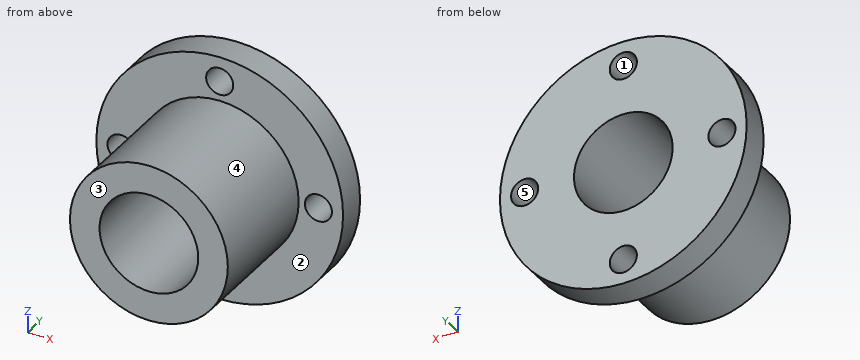
```python
from build123d import *

# Parameters (mm, degrees)
F0_R     = 25
F1_DEPTH = 6
F2_R     = 16
F3_DEPTH = 25
F4_R     = 2.75
F5_DEPTH = 31.001
F7_D     = 20


with BuildPart() as f1:
    # F0 (on Front) → F1 (new body)
    with BuildSketch(Plane.XZ):
        Circle(F0_R)
    extrude(amount=F1_DEPTH)

    # F2 (on face) → F3 (join)
    with BuildSketch(Plane.XZ.offset(6)):
        Circle(F2_R)
    extrude(amount=F3_DEPTH)

    # F4 (on face) → F5 (cut, through all)
    with BuildSketch(Plane(origin=(0, 0, 0), x_dir=(-1, 0, 0), z_dir=(0, 1, 0))):
        with Locations((0, 20)):
            Circle(F4_R)
        with Locations((-20, 0)):
            Circle(F4_R)
        with Locations((20, 0)):
            Circle(F4_R)
        with Locations((0, -20)):
            Circle(F4_R)
    extrude(amount=-F5_DEPTH, mode=Mode.SUBTRACT)

    # F7 (through all)
    with Locations(Plane(origin=(0, 0, 0), x_dir=(-1, 0, 0), z_dir=(0, 1, 0))):
        with Locations((0, 0)):
            Hole(F7_D / 2)


solid = f1.part
```
CAD build for the part. Positions are in the model's coordinates, mm. Face numbers are marked on the shaded views. A direction names the side the tool comes from. Coordinates: 2 decimals unless noted, no trailing zeros. Order: outer loops, then holes, each group sorted by start corner. A loop starts at its lowest first (then second) coordinate and runs counter-clockwise, first axis right, second up. Notation, with made-up numbers: M 27,51.5 L 43,51.5 A12 ccw 43,69.5 Z; hole C 33.25,-21.5 d10. An arc over 180 degrees is marked long. Answer as CSV lines item,"result".
1) Flat gauge pins, fed straight in: P1, Ø3, axis at y = -3.5, z = 8, coming from the -X side; P2, Ø8, axis at x = -2, y = -14.5, coming from the -Z side; P3, Ø6, axis at x = 17, y = -25.5, coming from the -Z side; P4, Ø4.5, axis at x = 0, z = -20, coming from the +Y side. Where does each tip first touch, or does it go through?
Verdict:
P1,"x = -24.14"
P2,"z = -16"
P3,"z = -7.75"
P4,"through"
2) Cut at B-B (x = -20). List the corners of the cut face in (y, z).
Verdict:
outline,"M -6,-15 L 0,-15 L 0,-2.75 L -6,-2.75 Z; M -6,2.75 L 0,2.75 L 0,15 L -6,15 Z"
3) Mould opens along Z. For the marked faces 3, 4 and 5 say: released by +Z, released by -Z, zero draft, split by the parting line, or undercut.
Verdict:
face 3,"zero draft"
face 4,"split by the parting line"
face 5,"undercut"
4) Drill centre lines: L1, parallel to Z at x = 0, y = -4.3; L2, parallel to Z at x = -2, y = -5.5; L3, parallel to Z at x = 0, y = -9. Where is each one in solid material? Low to high. Write a range as from..to.
Verdict:
L1,"-25..-22.75, -17.25..-10, 10..17.25, 22.75..25"
L2,"-24.92..-21.89, -18.11..-9.8, 9.8..18.11, 21.89..24.92"
L3,"-16..-10, 10..16"
5) Cut at D-D (x = 0). List the corners of the cut face in (y, z), then the cut area to 3 significant figures.
Verdict:
outline,"M -31,-16 L -6,-16 L -6,-17.25 L 0,-17.25 L 0,-10 L -31,-10 Z; M -31,10 L 0,10 L 0,17.25 L -6,17.25 L -6,16 L -31,16 Z; M -6,-25 L 0,-25 L 0,-22.75 L -6,-22.75 Z; M -6,22.75 L 0,22.75 L 0,25 L -6,25 Z"
area,"414 mm2"
6) Cut at A-A (z = 20). List the corners of the cut face in (x, y), then the cut area to 3 significant figures.
Verdict:
outline,"M -15,-6 L -2.75,-6 L -2.75,0 L -15,0 Z; M 2.75,-6 L 15,-6 L 15,0 L 2.75,0 Z"
area,"147 mm2"
7) 3-axis set-ups, long thin cutter, end or side, ignore diameter. For the marked faces 1 and 2: which of +Z, -Z, +X, -X, +Y, -Y reach the whole face in a straight line?
Verdict:
face 1,"+Y, -Y"
face 2,"-Y"
8) Cut at C-C (z = 0). List the corners of the cut face in (x, y).
Verdict:
outline,"M -25,-6 L -22.75,-6 L -22.75,0 L -25,0 Z; M -17.25,-6 L -16,-6 L -16,-31 L -10,-31 L -10,0 L -17.25,0 Z; M 10,-31 L 16,-31 L 16,-6 L 17.25,-6 L 17.25,0 L 10,0 Z; M 22.75,-6 L 25,-6 L 25,0 L 22.75,0 Z"
